```python
from build123d import *

# Parameters (mm, degrees)
SKETCH2_R               = 4.25
CUT_EXTRUDE1_DEPTH      = 15.666678844
CUT_EXTRUDE1_DEPTH_BACK = 10
SKETCH3_R               = 4.25
CUT_EXTRUDE2_DEPTH      = 15.666678844
CUT_EXTRUDE2_DEPTH_BACK = 10
CHAMFER1_SIZE           = 10
CHAMFER1_SIZE2          = 0.174550649
CHAMFER1_PART_2_SIZE    = 10
CHAMFER1_PART_2_SIZE2   = 0.174550649
SKETCH4_OUTSIDE_W       = 54.998
SKETCH4_OUTSIDE_H       = 54.998
SKETCH4_OUTSIDE_W_2     = 32
SKETCH4_OUTSIDE_H_2     = 40
CUT_EXTRUDE3_DEPTH      = 33
SKETCH5_R               = 50
BOSS_EXTRUDE1_DEPTH     = 10
SKETCH6_R               = 50
BOSS_EXTRUDE2_DEPTH     = 10


with BuildPart() as part:
    # Sketch1 → Revolve2 (revolve)
    with BuildSketch(Plane(origin=(0, 0, 0), x_dir=(0, 0, -1), z_dir=(1, 0, 0))):
        with BuildLine():
            Line((0, 12), (16, 12))
            ThreePointArc((16, 12), (17.88854382, -8.94427191), (0, -20))
            Line((0, -20), (0, 12))
        make_face()
    revolve(axis=Axis((0, -20, 0), (0, 1, 0)))

    # Sketch2 → Cut-Extrude1 (cut, two sides)
    with BuildSketch(Plane(origin=(0, 0, 0), x_dir=(0, 0, 1), z_dir=(0.139173101, 0.990268069, 0))) as cut_extrude1_sk:
        with Locations((0, 8)):
            Circle(SKETCH2_R)
    extrude(amount=CUT_EXTRUDE1_DEPTH, mode=Mode.SUBTRACT)
    extrude(cut_extrude1_sk.sketch, amount=-CUT_EXTRUDE1_DEPTH_BACK, mode=Mode.SUBTRACT)

    # Sketch3 → Cut-Extrude2 (cut, two sides)
    with BuildSketch(Plane(origin=(0, 0, 0), x_dir=(0, 0, 1), z_dir=(-0.139173101, 0.990268069, 0))) as cut_extrude2_sk:
        with Locations((0, -8)):
            Circle(SKETCH3_R)
    extrude(amount=CUT_EXTRUDE2_DEPTH, mode=Mode.SUBTRACT)
    extrude(cut_extrude2_sk.sketch, amount=-CUT_EXTRUDE2_DEPTH_BACK, mode=Mode.SUBTRACT)

    # Chamfer1
    chamfer1_edges = [part.edges().sort_by_distance(p)[0] for p in [
        (-6.53041354, -11.016065495, -4.25),
    ]]
    chamfer1_side = [part.faces().sort_by_distance(p)[0] for p in [
        (-8.197713558, 0.847390567, -4.25),
    ]]
    chamfer(chamfer1_edges, length=CHAMFER1_SIZE, length2=CHAMFER1_SIZE2, reference=chamfer1_side[0])

    # Chamfer1 part 2
    chamfer1_part_2_edges = [part.edges().sort_by_distance(p)[0] for p in [
        (6.53041354, -11.016065495, -4.25),
    ]]
    chamfer1_part_2_side = [part.faces().sort_by_distance(p)[0] for p in [
        (8.197713558, 0.847390567, -4.25),
    ]]
    chamfer(chamfer1_part_2_edges, length=CHAMFER1_PART_2_SIZE, length2=CHAMFER1_PART_2_SIZE2, reference=chamfer1_part_2_side[0])

    # Sketch4 outside → Cut-Extrude3 (cut, through all)
    with BuildSketch(Plane(origin=(0, 12, 0), x_dir=(1, 0, 0), z_dir=(0, 1, 0))):
        Rectangle(SKETCH4_OUTSIDE_W, SKETCH4_OUTSIDE_H)
        Rectangle(SKETCH4_OUTSIDE_W_2, SKETCH4_OUTSIDE_H_2, mode=Mode.SUBTRACT)
    extrude(amount=-CUT_EXTRUDE3_DEPTH, mode=Mode.SUBTRACT)

    # Sketch5 → Boss-Extrude1 (add)
    with BuildSketch(Plane(origin=(-16, 0, -32), x_dir=(0, 0, -1), z_dir=(1, 0, 0))):
        with Locations((-32, 0)):
            Circle(SKETCH5_R)
    extrude(amount=-BOSS_EXTRUDE1_DEPTH)

    # Sketch6 → Boss-Extrude2 (add)
    with BuildSketch(Plane(origin=(16, 0, 32), x_dir=(0, 0, 1), z_dir=(-1, 0, 0))):
        with Locations((-32, 0)):
            Circle(SKETCH6_R)
    extrude(amount=-BOSS_EXTRUDE2_DEPTH)


solid = part.part
```
Check sheet for the modelled part. Datum: model origin and axes. Units: mm. A direction names the side the tool comes from. Round coordinates to 2 decimals unless told otherwise and drop trailing zeros. Loops run counter-clockwise (first coordinate to the right, second up) from the corner with the lowest first, then second, coordinate; pieces in that order, holes last. Notation, with made-up numbers: (88, 24.25) - (141, 24.25) arc R27 cw to (141, 50.25) - close; hole circle Ø7 at (-8.75, 7). An arc over 180 degrees is marked (long way). Answer as a JSON object with one key per item and string values. Group by question number.
Q1. Sectioned sample at A-A, the plane z = 12. Enter the section's corners in (x, y).
Q2. Sectioned sample at B-B, the plane y = -34. Enter the section's corners in (x, z), plus the area to 3 significant figures.
Q3. Sectioned sample at C-C, the plane z = -37. Enter the section's corners in (x, y), plus the area to 3 significant figures.
Q4. Mould release check, pull along Y, two halves, no side actions. Record for faces 4 (the face through (-26, 1, 1)), 5 (the face through (6.587, -11.024, -0.057)), 6 (the face through (-20.93, 15.02, -47.69)): released by +Y, released by -Y, zero draft, split by the parting line, or undercut.
Q5. Set-up check for faces 1 (the face through (16, -10, 10)), 2 (the face through (26, 1, -1)), 3 (the face through (0, 12, 0)): record each of +Z, -Z, +X, -X, +Y, -Y from which the full face is reachable in a straight line by a thin tool's end or side.
Q6. Scan lines: line 1 along X through (y, z) = (-39, 2); line 2 along X through (y, z) = (-6, 16); line 3 along Y through (x, z) = (18, -41). Record each from-to range of solid material in increasing order. Write a range as [from, to].
Q7. Gauge pin test, flat end, axial feed: P1, Ø5, axis at x = 7, z = -5, coming from the +Y side. Record the tip position at first contact, or that the pin passes through.
Q8. Sectioned sample at D-D, the plane z = -9. Enter the section's corners in (x, y).
Solution:
{
 "1": {"outline": "(-26, -48.54) - (-16, -48.54) - (-16, 48.54) - (-26, 48.54) - close; (-10.58, 12) arc R16 ccw (long way) to (10.58, 12) - close; (16, -48.54) - (26, -48.54) - (26, 48.54) - (16, 48.54) - close"},
 "2": {"outline": "(-26, -36.66) - (-16, -36.66) - (-16, 36.66) - (-26, 36.66) - close; (16, -36.66) - (26, -36.66) - (26, 36.66) - (16, 36.66) - close", "area": "1,470 mm²"},
 "3": {"outline": "(-26, -33.63) - (-16, -33.63) - (-16, 33.63) - (-26, 33.63) - close; (16, -33.63) - (26, -33.63) - (26, 33.63) - (16, 33.63) - close", "area": "1,350 mm²"},
 "4": {"face 4": "zero draft", "face 5": "undercut", "face 6": "split by the parting line"},
 "5": {"face 1": "none", "face 2": "+Z, -Z, +X, +Y, -Y", "face 3": "+Z, -Z, +Y"},
 "6": {"line 1": "x = [-26, -16], [16, 26]", "line 2": "x = [-26, -16], [-10.39, 10.39], [16, 26]", "line 3": "y = [-28.62, 28.62]"},
 "7": {"P1": "stops at y = 12"},
 "8": {"outline": "(-26, -49.18) - (-16, -49.18) - (-16, -7.94) arc R17.86 ccw to (16, -7.94) - (16, -49.18) - (26, -49.18) - (26, 49.18) - (16, 49.18) - (16, 7.94) arc R17.86 ccw to (13.23, 12) - (-13.23, 12) arc R17.86 ccw to (-16, 7.94) - (-16, 49.18) - (-26, 49.18) - close"}
}
